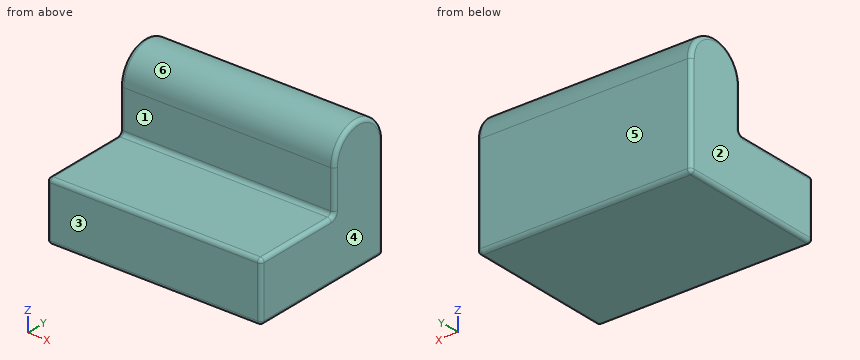
from build123d import *

# Parameters (mm, degrees)
F1_DEPTH = 709.6125
F2_R     = 25.4
F3_SCALE = 0.05


with BuildPart() as f1:
    # F0 (on Right) → F1 (new body, symmetric)
    with BuildSketch(Plane.YZ):
        with BuildLine():
            Line((-1000.125, 0), (0, 0))
            Line((0, 0), (0, 669.925))
            ThreePointArc((0, 669.925), (-200.025, 869.95), (-400.05, 669.925))
            Line((-400.05, 669.925), (-400.05, 390.525))
            Line((-400.05, 390.525), (-1000.125, 390.525))
            Line((-1000.125, 390.525), (-1000.125, 0))
        make_face()
    extrude(amount=F1_DEPTH, both=True)

    # F2
    f2_edges = [f1.edges().sort_by_distance(p)[0] for p in [
        (709.6125, 0, 334.9625),
        (-709.6125, -500.0625, 0),
        (0, 0, 0),
        (709.6125, -500.0625, 0),
        (0, -1000.125, 0),
        (-709.6125, 0, 334.9625),
        (-709.6125, -200.025, 869.95),
        (-709.6125, -400.05, 530.225),
        (-709.6125, -700.0875, 390.525),
        (-709.6125, -1000.125, 195.2625),
        (0, -1000.125, 390.525),
        (709.6125, -200.025, 869.95),
        (709.6125, -400.05, 530.225),
        (709.6125, -700.0875, 390.525),
        (709.6125, -1000.125, 195.2625),
        (0, -400.05, 390.525),
        (0, -400.05, 669.925),
        (0, 0, 669.925),
    ]]
    fillet(f2_edges, radius=F2_R)


with BuildPart() as f1_1:
    # F3: moved
    add(f1.part.scale(F3_SCALE))


solid = f1_1.part
Design review of the part built by this model. Coordinates are the model's own, in mm. Face numbers are marked on the shaded views. A direction names the side the tool comes from. Coordinates: 2 decimals unless noted, no trailing zeros. Write each loop counter-clockwise with the first axis right and the second up, starting at its lowest first coordinate (ties: lowest second). Pieces come first, ordered by that corner, then holes. Notation, with made-up numbers: (35, -10.5) -> (49, -10.5) arc R22 ccw to (49, 10.5) -> close; hole circle Ø5 at (72.25, -4.75). An arc over 180 degrees is marked (long way). Write each question's results on one line, items separated by ' | '. Start each with the question number.
(1) For line 1 along Z through (x, y) = (-22, -41); line 2 along Y through (x, z) = (-20.5, 30); line 3 along Z through (x, y) = (20.5, -7), list the stretches that pass through material, from the lowest coordinate up. Write a range as from..to.
(2) Tool access review of the marked faces 1 and 2: name each direction out of +Z, -Z, +X, -X, +Y, -Y from which nothing blocks a thin tool from reaching the whole face with its end or side.
(3) Take a section at C-C on z = 23. Write out the cut boundary in (x, y), and give its area (3 significant figures).
(4) Take a section at A-A on y = -39. Write out the cut boundary in (x, z).
(5) The part is to be moulded in two halves that separate along Y. For the marked faces 3, 4, 5 and 6, say which applies: pulls with the +Y half, pulls with the -Y half, needs draft (parallel to the pull), parting line crosses it, or undercut.
(6) Clearance check with flat-ended pins moving along their axes: P1, Ø2, axis at x = 26, y = -15.5, coming from the +Z side; P2, Ø3, axis at x = -5, y = -38.5, coming from the +Z side; P3, Ø5, axis at x = -13.5, z = 37.5, coming from the -Y side. State where each tip first meets the part, or that it passes through.
(7) Take a section at B-B on x = 10. Write out the cut boundary in (y, z).
Results found:
1) line 1: z = 0..19.53 | line 2: y = -20..0 | line 3: z = 0..43.04
2) face 1: +Z, +X, -X, -Y | face 2: +Z, -Z, -X, +Y, -Y
3) outline: (-35.48, -18.73) arc R1.27 ccw to (-34.21, -20) -> (34.21, -20) arc R1.27 ccw to (35.48, -18.73) -> (35.48, -1.27) arc R1.27 ccw to (34.21, 0) -> (-34.21, 0) arc R1.27 ccw to (-35.48, -1.27) -> close | area: 1,420 mm2
4) outline: (-35.48, 1.27) arc R1.27 ccw to (-34.21, 0) -> (34.21, 0) arc R1.27 ccw to (35.48, 1.27) -> (35.48, 18.26) arc R1.27 ccw to (34.21, 19.53) -> (-34.21, 19.53) arc R1.27 ccw to (-35.48, 18.26) -> close
5) face 3: pulls with the -Y half | face 4: needs draft | face 5: pulls with the +Y half | face 6: parting line crosses it
6) P1: stops at z = 42.43 | P2: stops at z = 19.53 | P3: stops at y = -19.89
7) outline: (-50.01, 1.27) arc R1.27 ccw to (-48.74, 0) -> (-1.27, 0) arc R1.27 ccw to (0, 1.27) -> (0, 33.5) arc R10 ccw to (-20, 33.5) -> (-20, 20.8) arc R1.27 cw to (-21.27, 19.53) -> (-48.74, 19.53) arc R1.27 ccw to (-50.01, 18.26) -> close
